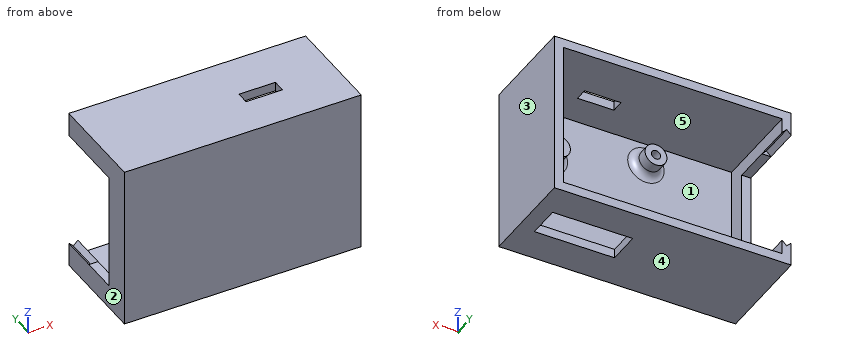
```python
from build123d import *

# Parameters (mm, degrees)
SKETCH_1_W          = 65
SKETCH_1_H          = 45
EXTRUDE_1_DEPTH     = 27.5
SHELL_1_T           = -2.5
SKETCH_3_W          = 32
SKETCH_3_H          = 20
CUT_EXTRUDE_1_DEPTH = 3.5
CUT_EXTRUDE_2_DEPTH = 10
SKETCH_5_R          = 3
SKETCH_5_R_2        = 1.25
EXTRUDE_2_DEPTH     = 5
SKETCH_6_R          = 3
SKETCH_6_R_2        = 0.75
EXTRUDE_3_DEPTH     = 5
SKETCH_7_W          = 22
SKETCH_7_H          = 9
CUT_EXTRUDE_3_DEPTH = 3.5
SKETCH_8_W          = 10
SKETCH_8_H          = 3.5
CUT_EXTRUDE_4_DEPTH = 3.5
FILLET_1_R          = 2


with BuildPart() as part:
    # 草图1 → 凸台-拉伸1 (new body)
    with BuildSketch(Plane(origin=(0, 0, 0), x_dir=(1, 0, 0), z_dir=(0, 1, 0))):
        Rectangle(SKETCH_1_W, SKETCH_1_H)
    extrude(amount=EXTRUDE_1_DEPTH)

    # 抽壳1
    shell_1_openings = [part.faces().sort_by_distance(p)[0] for p in [
        (0, 27.5, 0),
    ]]
    offset(amount=SHELL_1_T, openings=shell_1_openings, kind=Kind.INTERSECTION)

    # 草图3 → 切除-拉伸1 (cut, through all)
    with BuildSketch(Plane(origin=(-30, 0, 0), x_dir=(0, 0, -1), z_dir=(1, 0, 0))):
        with Locations((0, 17.5)):
            Rectangle(SKETCH_3_W, SKETCH_3_H)
    extrude(amount=-CUT_EXTRUDE_1_DEPTH, mode=Mode.SUBTRACT)

    # 草图4 → 切除-拉伸2 (cut)
    with BuildSketch(Plane(origin=(0, 27.5, 0), x_dir=(1, 0, 0), z_dir=(0, 1, 0))):
        Polygon((-32.5, 16), (-31.25, 17.25), (-30, 16), align=None)
        Polygon((-32.5, -16), (-30, -16), (-31.25, -17.25), align=None)
    extrude(amount=-CUT_EXTRUDE_2_DEPTH, mode=Mode.SUBTRACT)

    # 草图5 → 凸台-拉伸2 (add)
    with BuildSketch(Plane(origin=(0, 2.5, 0), x_dir=(1, 0, 0), z_dir=(0, 1, 0))):
        with Locations((-6.5, 13.75)):
            Circle(SKETCH_5_R)
        with Locations((-6.5, 13.75)):
            Circle(SKETCH_5_R_2, mode=Mode.SUBTRACT)
        with Locations((-6.5, -13.75)):
            Circle(SKETCH_5_R)
        with Locations((-6.5, -13.75)):
            Circle(SKETCH_5_R_2, mode=Mode.SUBTRACT)
    extrude(amount=EXTRUDE_2_DEPTH)

    # 草图6 → 凸台-拉伸3 (add)
    with BuildSketch(Plane(origin=(0, 2.5, 0), x_dir=(1, 0, 0), z_dir=(0, 1, 0))):
        with Locations((20, -7)):
            Circle(SKETCH_6_R)
        with Locations((20, -7)):
            Circle(SKETCH_6_R_2, mode=Mode.SUBTRACT)
    extrude(amount=EXTRUDE_3_DEPTH)

    # 草图7 → 切除-拉伸3 (cut, through all)
    with BuildSketch(Plane.XY.offset(-20)):
        with Locations((17, 14)):
            Rectangle(SKETCH_7_W, SKETCH_7_H)
    extrude(amount=-CUT_EXTRUDE_3_DEPTH, mode=Mode.SUBTRACT)

    # 草图8 → 切除-拉伸4 (cut, through all)
    with BuildSketch(Plane(origin=(0, 0, 20), x_dir=(-1, 0, 0), z_dir=(0, 0, -1))):
        with Locations((-12, 12.75)):
            Rectangle(SKETCH_8_W, SKETCH_8_H)
    extrude(amount=-CUT_EXTRUDE_4_DEPTH, mode=Mode.SUBTRACT)

    # 圆角1
    fillet_1_edges = [part.edges().sort_by_distance(p)[0] for p in [
        (-9.5, 2.5, -13.75),
        (-9.5, 2.5, 13.75),
        (17, 2.5, 7),
    ]]
    fillet(fillet_1_edges, radius=FILLET_1_R)


solid = part.part
```
For this review, take the finished solid that the model builds, in its own axes (mm). Face numbers are marked on the shaded views. A direction names the side the tool comes from. Round coordinates to 2 decimals unless told otherwise and drop trailing zeros. Write each loop counter-clockwise with the first axis right and the second up, starting at its lowest first coordinate (ties: lowest second). Pieces come first, ordered by that corner, then holes. Notation, with made-up numbers: (-17.5, 13) -> (18.5, 13) arc R27 ccw to (18.5, 46) -> close; hole circle Ø8 at (82, 67). An arc over 180 degrees is marked (long way). One line per question, with ' | ' between items. Start each with the question number.
(1) Mouldability with a two-part tool opening along X and no side actions: class the marked faces 3, 4 and 5 as released by +X, released by -X, zero draft, split by the parting line, or undercut.
(2) For line 1 along X through (y, z) = (5.15, 7); line 2 along Z through (x, y) = (20, 6.45); line 3 along X through (y, z) = (5.65, 13.75), list the stretches that pass through material, from the lowest coordinate up. Write a range as from..to.
(3) Add section A-A, the plane y = 16.75. Write out the cut boundary in (x, z), plus the area to 3 significant figures.
(4) Add section B-B, the plane x = 20. Write out the cut boundary in (y, z), plus the area to 3 significant figures.
(5) Add section D-D, the plane x = -17.5. Write out the cut boundary in (y, z).
(6) Insertion check: P1, Ø5, axis at x = -7.5, z = 12.5, coming from the +Y side; P2, Ø6, axis at y = 14, z = -1.5, coming from the -X side; P3, Ø12, axis at x = -1.5, z = -1.5, coming from the +Y side. Each pin has a flat end and moves straight along its axis. Give the tip position at first contact, or say it passes through.
(7) Tool access review of the marked faces 1 and 2: name each direction out of +Z, -Z, +X, -X, +Y, -Y from which nothing blocks a thin tool from reaching the whole face with its end or side.
(8) Add section C-C, the plane z = -13.75. Write out the cut boundary in (x, y), plus the area to 3 significant figures.
Answer list:
1) face 3: released by +X | face 4: zero draft | face 5: undercut
2) line 1: -32.5..-30, 17..19.25, 20.75..23, 30..32.5 | line 2: -22.5..-20, 4..6.25, 7.75..10, 20..22.5 | line 3: -32.5..-30, -9.5..-7.75, -5.25..-3.5, 30..32.5
3) outline: (-32.5, -22.5) -> (6, -22.5) -> (6, -20) -> (-30, -20) -> (-30, -16) -> (-32.5, -16) -> close; (-32.5, 16) -> (-30, 16) -> (-30, 20) -> (30, 20) -> (30, -20) -> (28, -20) -> (28, -22.5) -> (32.5, -22.5) -> (32.5, 22.5) -> (-32.5, 22.5) -> close | area: 390 mm²
4) outline: (0, -22.5) -> (9.5, -22.5) -> (9.5, -20) -> (2.5, -20) -> (2.5, 2) arc R2 cw to (4.5, 4) -> (7.5, 4) -> (7.5, 6.25) -> (2.5, 6.25) -> (2.5, 7.75) -> (7.5, 7.75) -> (7.5, 10) -> (4.5, 10) arc R2 cw to (2.5, 12) -> (2.5, 20) -> (27.5, 20) -> (27.5, 22.5) -> (0, 22.5) -> close; (18.5, -22.5) -> (27.5, -22.5) -> (27.5, -20) -> (18.5, -20) -> close | area: 239 mm²
5) outline: (0, -22.5) -> (27.5, -22.5) -> (27.5, -20) -> (2.5, -20) -> (2.5, 20) -> (27.5, 20) -> (27.5, 22.5) -> (0, 22.5) -> close
6) P1: y = 7.5 | P2: x = 30 | P3: y = 2.5
7) face 1: +Y | face 2: +Z, -Z, -X, +Y, -Y
8) outline: (-32.5, 0) -> (32.5, 0) -> (32.5, 27.5) -> (30, 27.5) -> (30, 2.5) -> (-1.5, 2.5) arc R2 cw to (-3.5, 4.5) -> (-3.5, 7.5) -> (-5.25, 7.5) -> (-5.25, 2.5) -> (-7.75, 2.5) -> (-7.75, 7.5) -> (-9.5, 7.5) -> (-9.5, 4.5) arc R2 cw to (-11.5, 2.5) -> (-30, 2.5) -> (-30, 7.5) -> (-32.5, 7.5) -> close | area: 257 mm²
